from build123d import *

# Parameters (mm, degrees)
F1_DEPTH = 25.4
F2_R     = 6.35
F3_DEPTH = 25.4


with BuildPart() as f1:
    # F0 (on Front) → F1 (new body)
    with BuildSketch(Plane.XZ):
        Polygon((-11.320572, 27.37729), (-29.535599, -2.306457), (-6.933432, -28.802758), (25.250503, -15.494627), (22.5391, 19.226552), align=None)
    extrude(amount=F1_DEPTH)

    # F2 (on face) → F3 (cut)
    with BuildSketch(Plane.XZ.offset(25.4)):
        Circle(F2_R)
    extrude(amount=-F3_DEPTH, mode=Mode.SUBTRACT)


solid = f1.part
Input: part model. Units: mm. Frame: model coordinates. Coordinates: 2 decimals unless noted, no trailing zeros. Order: outer loops, then holes, each group sorted by start corner. A loop starts at its lowest first (then second) coordinate and runs counter-clockwise, first axis right, second up. Notation, with made-up numbers: M 42.25,12.5 L 82.25,12.5 A21 cw 82.25,28.5 Z; hole C -31,8.5 d8. An arc over 180 degrees is marked long. Answer in a Markdown table with one row per item.
(1) Section query A-A, the plane y = -1.25. Output: boundary loops of the cut face in (x, z), plus the area to 3 significant figures.
Numbers:
| item | result |
|---|---|
| outline | M -29.54,-2.31 L -6.93,-28.8 L 25.25,-15.49 L 22.54,19.23 L -11.32,27.38 Z; hole C 0,0 d12.7 |
| area | 1,960 mm^2 |
(2) Section query B-B, the plane z = 0. Output: boundary loops of the cut face in (x, y).
Numbers:
| item | result |
|---|---|
| outline | M -28.12,-25.4 L -6.35,-25.4 L -6.35,0 L -28.12,0 Z; M 6.35,-25.4 L 24.04,-25.4 L 24.04,0 L 6.35,0 Z |
(3) Contact query for flat-ended pins moving along their axis: pin 1 Ø8 at (y, z) = (-6, 5) entering from +X; pin 2 Ø1.5 at (x, y) = (13, -5.5) entering from -Z; pin 3 Ø6 at (x, y) = (14, -15) entering from +Z; pin 4 Ø10 at (x, z) = (0, 0) entering from +Y. Output: stop coordinate, or through.
Numbers:
| item | result |
|---|---|
| pin 1 | stops at x = 23.96 |
| pin 2 | stops at z = -20.87 |
| pin 3 | stops at z = 22 |
| pin 4 | passes through |
(4) Material intervals for line 1 (Z direction, x = 0, y = -5); line 2 (Z direction, x = -1, y = -8.5); line 3 (X direction, y = -23.5, z = 8), sorted ascending. Write a range as [from, to].
Numbers:
| item | result |
|---|---|
| line 1 | z = [-25.94, -6.35], [6.35, 24.65] |
| line 2 | z = [-26.35, -6.27], [6.27, 24.89] |
| line 3 | x = [-23.21, 23.42] |
(5) Draft query along Z for faces 1 (the flat face through (4, -25.4, 6)), 2 (the cylindrical face through (-1.38, -12.88, -6.2)), 3 (the flat face through (23.914, -12.522, 1.623)), 4 (the flat face through (8.933, -12.522, -22.242)). Return one class per face: pulls with the +Z half, pulls with the -Z half, needs draft (parallel to the pull), parting line crosses it, or undercut.
Numbers:
| item | result |
|---|---|
| face 1 | needs draft |
| face 2 | undercut |
| face 3 | pulls with the +Z half |
| face 4 | pulls with the -Z half |
(6) Section query D-D, the plane x = 21. Output: boundary loops of the cut face in (y, z), plus the area to 3 significant figures.
Numbers:
| item | result |
|---|---|
| outline | M -25.4,-17.25 L 0,-17.25 L 0,19.6 L -25.4,19.6 Z |
| area | 936 mm^2 |
(7) Section query C-C, the plane x = -2.5. Output: boundary loops of the cut face in (y, z), plus the area to 3 significant figures.
Numbers:
| item | result |
|---|---|
| outline | M -25.4,-26.97 L 0,-26.97 L 0,-5.84 L -25.4,-5.84 Z; M -25.4,5.84 L 0,5.84 L 0,25.25 L -25.4,25.25 Z |
| area | 1,030 mm^2 |
